Autodesk Inventor part; units mm, degrees
ref_plane "YZ Plane" through (0, 0, 0) normal (1, 0, 0) x (0, 1, 0)
ref_plane "XZ Plane" through (0, 0, 0) normal (0, 1, 0) x (-1, 0, 0)
ref_plane "XY Plane" through (0, 0, 0) normal (0, 0, 1) x (1, 0, 0)
sketch "Sketch8" plane through (0, 0, 0) normal (0, 0, 1) x (1, 0, 0)
  line L0 (-25, 20) -> (25, 20)
  line L1 (30, 15) -> (30, -15)
  line L2 (25, -20) -> (-25, -20)
  line L3 (-30, -15) -> (-30, 15)
  line L4 (-30, 20) -> (30, -20) construction
  line L5 (30, 20) -> (-30, -20) construction
  line L6 (-25, 15) -> (25, 15) construction
  line L7 (25, 15) -> (25, -15) construction
  line L8 (25, -15) -> (-25, -15) construction
  line L9 (-25, -15) -> (-25, 15) construction
  line L10 (-25, 15) -> (25, -15) construction
  line L11 (25, 15) -> (-25, -15) construction
  circle A0 centre (-25, 15) radius 2
  circle A1 centre (25, 15) radius 2
  circle A2 centre (25, -15) radius 2
  circle A3 centre (-25, -15) radius 2
  arc A4 (-25, 20) -> (-30, 15) centre (-25, 15) ccw
  arc A5 (-30, -15) -> (-25, -20) centre (-25, -15) ccw
  arc A6 (25, -20) -> (30, -15) centre (25, -15) ccw
  arc A7 (30, 15) -> (25, 20) centre (25, 15) ccw
  point P0 (0, 0)
  dimension "d30" = 40
  dimension "d31" = 4
  dimension "d32" = 50
  dimension "d33" = 60
  dimension "d34" = 30
  dimension "d35" = 5
extrude "Extrusion8" add sketch "Sketch8" along normal blind 5
sketch "Sketch9" plane through (0, 0, 5) normal (0, 0, 1) x (1, 0, 0)
  line L0 (-25, -20) -> (25, -20)
  line L1 (-18, 20) -> (-6, 20)
  line L2 (-6, 20) -> (-6, -20)
  line L3 (-6, -20) -> (-18, -20)
  line L4 (-18, -20) -> (-18, 20)
  line L5 (-18, 20) -> (-6, -20) construction
  line L6 (-6, 20) -> (-18, -20) construction
  line L7 (6, 20) -> (18, 20)
  line L8 (18, 20) -> (18, -20)
  line L9 (18, -20) -> (6, -20)
  line L10 (6, -20) -> (6, 20)
  line L11 (6, 20) -> (18, -20) construction
  line L12 (18, 20) -> (6, -20) construction
  line L13 (25, 20) -> (-25, 20)
  point P0 (0, 0)
  point P1 (-12, 0)
  point P2 (12, 0)
  dimension "d38" = 12
  dimension "d39" = 6
  dimension "d40" = 6
extrude "Extrusion9" add sketch "Sketch9" along normal blind 40 contours L4 L1 L2 L0 | L10 L7 L8 L0
fillet "Fillet3" radius 5 2 edges at (-18, 0, 5) (18, 0, 5)
sketch "Sketch10" plane through (18, -20, 45) normal (1, 0, 0) x (0, 0, -1)
  circle A0 centre (20, 20) radius 8.5
  circle A1 centre (20, 20) radius 20
  line L0 (0, 0) -> (0, 40)
  line L1 (38.3283, 0) -> (41.7977, 39.6968)
  line L2 (20, 0) -> (0, 0)
  line L3 (20, 0) -> (0, 0)
  line L4 (0, 0) -> (0, 40)
  line L5 (0, 40) -> (20, 40)
  line L6 (35, 40) -> (0, 40)
  line L7 (0, 0) -> (0, 40)
  line L8 (35, 0) -> (0, 0)
  point P0 (45, 20)
  point P1 (45, 20)
  point P2 (0, 20)
  dimension "d44" = 17
extrude "Extrusion10" cut sketch "Sketch10" against normal through all contours A0 | A1 L0 L5 | A1 L2 L0
sketch "Sketch5" plane through (0, 0, 0) normal (0, 0, 1) x (1, 0, 0)
  line L0 (15, 15) -> (15, -15) construction
  line L1 (15, -15) -> (-15, -15) construction
  line L2 (-15, -15) -> (-15, 15) construction
  line L3 (-15, 15) -> (15, -15) construction
  line L4 (15, 15) -> (-15, -15) construction
  circle A0 centre (-15, 15) radius 2
  circle A1 centre (15, 15) radius 2
  circle A2 centre (15, -15) radius 2
  circle A3 centre (-15, -15) radius 2
  line L5 (-15, 20) -> (15, 20)
  line L6 (20, 15) -> (20, -15)
  line L7 (15, -20) -> (-15, -20)
  line L8 (-20, -15) -> (-20, 15)
  line L9 (-20, 20) -> (20, -20) construction
  line L10 (20, 20) -> (-20, -20) construction
  arc A4 (20, 15) -> (15, 20) centre (15, 15) ccw
  arc A5 (15, -20) -> (20, -15) centre (15, -15) ccw
  arc A6 (-20, -15) -> (-15, -20) centre (-15, -15) ccw
  arc A7 (-15, 20) -> (-20, 15) centre (-15, 15) ccw
  point P0 (0, 0)
  dimension "d16" = 4
  dimension "d17" = 30
  dimension "d18" = 40
  dimension "d20" = 5
sketch "Sketch6" plane through (0, 0, 10) normal (0, 0, 1) x (1, 0, 0)
  line L0 (-15, -20) -> (15, -20)
  line L1 (-6, 20) -> (6, 20)
  line L2 (6, 20) -> (6, -20)
  line L3 (6, -20) -> (-6, -20)
  line L4 (-6, -20) -> (-6, 20)
  line L5 (-6, 20) -> (6, -20) construction
  line L6 (6, 20) -> (-6, -20) construction
  point P0 (0, 0)
  dimension "d23" = 12
sketch "Sketch7" plane through (6, -20, 50) normal (1, 0, 0) x (0, 0, -1)
  circle A0 centre (20, 20) radius 8.5
  circle A1 centre (20, 20) radius 20
  line L0 (0, 0) -> (0, 40)
  line L1 (40, 0) -> (40, 40)
  line L2 (35, 0) -> (0, 0)
  line L3 (20, 0) -> (0, 0)
  line L4 (0, 0) -> (0, 40)
  line L5 (0, 40) -> (20, 40)
  line L6 (35, 40) -> (0, 40)
  point P0 (50, 20)
  point P1 (0, 20)
  dimension "d27" = 17
sketch "Sketch1" plane through (0, 0, 0) normal (0, 1, 0) x (-1, 0, 0)
  line L0 (27.5, 22.5) -> (-27.5, 22.5)
  line L1 (-27.5, 22.5) -> (-27.5, -22.5)
  line L2 (-27.5, -22.5) -> (27.5, -22.5)
  line L3 (27.5, -22.5) -> (27.5, 22.5)
  point P0 (0, 0)
  point P1 (27.5, 0)
  point P2 (0, -22.5)
  dimension "d0" = 45
  dimension "d1" = 55
sketch "Sketch2" plane through (0, 10, 0) normal (0, 1, 0) x (1, 0, 0)
  line L0 (-27.5, 22.5) -> (-27.5, -22.5)
  line L1 (-27.5, -22.5) -> (27.5, -22.5)
  line L2 (-27.5, 22.5) -> (-19.5, 22.5)
  line L3 (-19.5, 22.5) -> (-19.5, -22.5)
  line L4 (-19.5, -22.5) -> (-27.5, -22.5)
  line L5 (-27.5, -22.5) -> (-27.5, 22.5)
  line L6 (27.5, -22.5) -> (27.5, 22.5)
  line L7 (27.5, 22.5) -> (19.5, 22.5)
  line L8 (19.5, 22.5) -> (19.5, -22.5)
  line L9 (19.5, -22.5) -> (27.5, -22.5)
  line L10 (27.5, -22.5) -> (27.5, 22.5)
  point P0 (0, 0)
  dimension "d4" = 8
  dimension "d5" = 8
sketch "Sketch4" plane through (0, 0, 0) normal (0, -1, 0) x (1, 0, 0)
  line L0 (15, 15) -> (-15, 15) construction
  line L1 (-15, 15) -> (-15, -15) construction
  line L2 (-15, -15) -> (15, -15) construction
  line L3 (15, -15) -> (15, 15) construction
  line L4 (15, 15) -> (-15, -15) construction
  line L5 (-15, 15) -> (15, -15) construction
  circle A0 centre (15, -15) radius 2
  circle A1 centre (-15, -15) radius 2
  circle A2 centre (-15, 15) radius 2
  circle A3 centre (15, 15) radius 2
  point P0 (0, 0)
  dimension "d12" = 30
  dimension "d13" = 4
sketch "Sketch3" plane through (27.5, 0, 22.5) normal (1, 0, 0) x (0, 0, -1)
  circle A0 centre (22.5, 25) radius 15
  line L0 (22.5, 25) -> (22.5, 47.5) construction
  line L1 (45, 47.5) -> (0, 47.5)
  line L2 (22.5, 25) -> (45, 25) construction
  line L3 (45, 0) -> (45, 47.5)
  point P0 (22.5, 0)
  dimension "d9" = 30
properties part number "DoubleHinge"
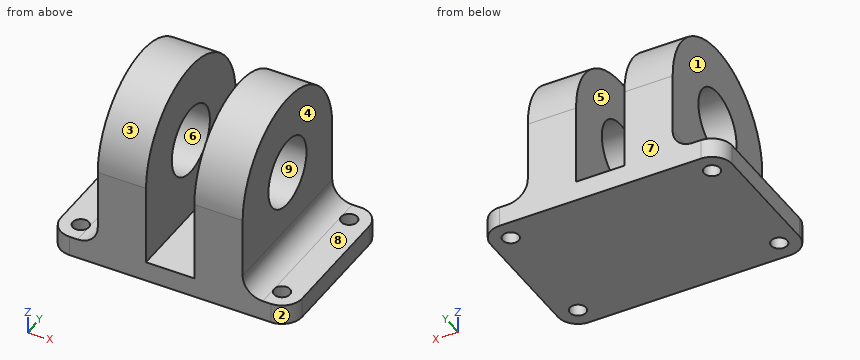
Work out the finished part from the listing and answer in its coordinate system (mm). Face numbers are marked on the shaded views. A direction names the side the tool comes from. Coordinates: 2 decimals unless noted, no trailing zeros. Write each loop counter-clockwise with the first axis right and the second up, starting at its lowest first coordinate (ties: lowest second). Pieces come first, ordered by that corner, then holes.
Q1. Determine the mould class of the marked faces 6, 7, 8 and 9 for opening direction Z: released by +Z, released by -Z, zero draft, split by the parting line, or undercut.
Q2. A cutting plane is placed at C-C, the plane z = 15. Give the vertices of the cut face in (x, y).
Q3. Find the intervals of material crossed by line 1 (Y direction, x = -25, z = 1.45); line 2 (X direction, y = -13.5, z = 24); line 3 (Y direction, x = -8, z = 25), in increasing order.
Q4. Which of the six approach directions +Z, -Z, +X, -X, +Y, -Y give full straight-line access (tool end or side, diameter ignored) to the marked faces 1, 2, 3, 4 and 5?
Q5. A cutting plane is placed at A-A, the plane z = 4. Give the vertices of the cut face in (x, y).
Q6. A cutting plane is placed at B-B, the plane y = -5. Give the vertices of the cut face in (x, z), then the cut area to 3 significant figures.
Q7. Each of these flat-tipped pins is pushed along its axis until it touches: pin 1 Ø3.5 at (x, y) = (25, 15) entering from +Z; pin 2 Ø10.5 at (y, z) = (-4.5, 24.5) entering from +X; pin 3 Ø6 at (y, z) = (9, 10) entering from +X; pin 4 Ø2 at (x, y) = (-26.5, 9.5) entering from +Z. Where does it stop, or does it pass through?
Q8. A cutting plane is placed at D-D, the plane x = 13.5. Give the vertices of the cut face in (y, z).
Findings below:
1. face 6: undercut
1. face 7: zero draft
1. face 8: released by +Z
1. face 9: undercut
2. outline: (-18, -20) - (-6, -20) - (-6, 20) - (-18, 20) - close; (6, -20) - (18, -20) - (18, 20) - (6, 20) - close
3. line 1: y = -20 to -17, -13 to 13, 17 to 20
3. line 2: x = -18 to -6, 6 to 18
3. line 3: y = -20 to -8.5, 8.5 to 20
4. face 1: +Z, -X, +Y, -Y
4. face 2: +Z, -Z, +X, -Y
4. face 3: +Z, +X, -X
4. face 4: +Z, +X, +Y, -Y
4. face 5: +Z, +Y, -Y
5. outline: (-30, -15) arc R5 ccw to (-25, -20) - (25, -20) arc R5 ccw to (30, -15) - (30, 15) arc R5 ccw to (25, 20) - (-25, 20) arc R5 ccw to (-30, 15) - close; hole circle Ø4 at (-25, -15); hole circle Ø4 at (-25, 15); hole circle Ø4 at (25, -15); hole circle Ø4 at (25, 15)
6. outline: (-30, 0) - (30, 0) - (30, 5) - (23, 5) arc R5 cw to (18, 10) - (18, 18.13) - (6, 18.13) - (6, 5) - (-6, 5) - (-6, 18.13) - (-18, 18.13) - (-18, 10) arc R5 cw to (-23, 5) - (-30, 5) - close; (-18, 31.87) - (-6, 31.87) - (-6, 44.36) - (-18, 44.36) - close; (6, 31.87) - (18, 31.87) - (18, 44.36) - (6, 44.36) - close
6. area: 926 mm2
7. pin 1: passes through
7. pin 2: stops at x = 18
7. pin 3: stops at x = 19
7. pin 4: stops at z = 5
8. outline: (-20, 0) - (20, 0) - (20, 25) arc R20 ccw to (-20, 25) - close; hole circle Ø17 at (0, 25)
